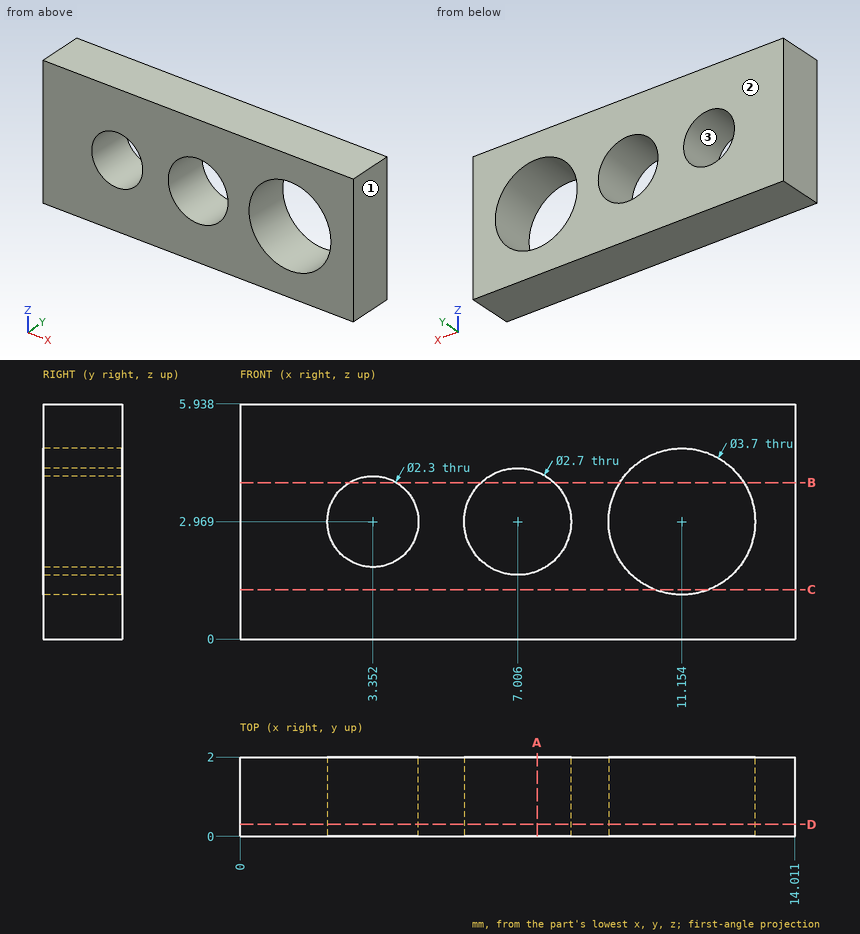
Study the drawing (mm; zero at the part's minimum x, y, z) and answer. Coordinates: 2 decimals unless noted, no trailing zeros. Order: outer loops, then holes, each group sorted by start corner. A loop starts at its lowest first (then second) coordinate and runs counter-clockwise, first axis right, second up. Notation, with made-up numbers: M -32,10 L 25,10 A13 ccw 25,19 Z; hole C 89,42 d2. An arc over 180 degrees is marked long. Answer as a JSON object with one key per item and string values. Group by question number.
1. Section A-A on x = 7.5 is taken. Write down the section's boundary in (y, z) (1 decimal).
2. Straight lines are drawn through the part: line 1 (X direction, y = 1.1, z = 2.9) (1 decimal); line 2 (Z direction, x = 11.25, y = 0.65); line 3 (X direction, y = 1.9, z = 3.7) (1 decimal). For each, find the intervals that lie inside material, in ascending order.
3. Section B-B on z = 3.95 is taken. Write down the section's boundary in (x, y) (1 decimal).
4. Section C-C on z = 1.25 is taken. Write down the section's boundary in (x, y), then the cut area to 3 significant figures.
5. Section D-D on y = 0.3 is taken. State how many separate pieces and enclosed holes the cut face has.
6. Determine the mould class of the marked faces 1, 2 and 3 for opening direction X: released by +X, released by -X, zero draft, split by the parting line, or undercut.
Values follow:
{
 "1": {"outline": "M 0,0 L 2,0 L 2,1.7 L 0,1.7 Z; M 0,4.2 L 2,4.2 L 2,5.9 L 0,5.9 Z"},
 "2": {"line 1": "0 to 2.2, 4.5 to 5.7, 8.4 to 9.3, 13 to 14", "line 2": "0 to 1.12, 4.82 to 5.94", "line 3": "0 to 2.5, 4.2 to 5.9, 8.1 to 9.5, 12.9 to 14"},
 "3": {"outline": "M 0,0 L 2.8,0 L 2.8,2 L 0,2 Z; M 4,0 L 6.1,0 L 6.1,2 L 4,2 Z; M 7.9,0 L 9.6,0 L 9.6,2 L 7.9,2 Z; M 12.7,0 L 14,0 L 14,2 L 12.7,2 Z"},
 "4": {"outline": "M 0,0 L 10.47,0 L 10.47,2 L 0,2 Z; M 11.84,0 L 14.01,0 L 14.01,2 L 11.84,2 Z", "area": "25.3 mm2"},
 "5": {"separate pieces": "1", "enclosed holes": "3"},
 "6": {"face 1": "released by +X", "face 2": "zero draft", "face 3": "undercut"}
}
